Read the model definition and answer for the solid it produces. Units are mm, in the model's axes. A direction names the side the tool comes from. Coordinates: 2 decimals unless noted, no trailing zeros. Write each loop counter-clockwise with the first axis right and the second up, starting at its lowest first coordinate (ties: lowest second). Pieces come first, ordered by that corner, then holes.
(1) Section C-C on x = -11 is taken. Write down the section's boundary in (y, z) (3 decimals), then the cut area to 3 significant figures.
(2) Given pin 1 (6 mm diameter, centred on x = -8.5, z = 97.5, fed in from +Y); pin 2 (6 mm diameter, centred on y = 5.5, z = 62.5, fed in from -X); pin 3 (12 mm diameter, centred on x = -9.5, y = 12, fed in from +Z), each flat-ended and moving along its own axis, determine where each tip first touches the part or whether it passes through.
(3) Find the intervals of material crossed by probe 1 along Y at (x, z) = (-12.25, 98); probe 2 along X at (y, z) = (25.5, 218), in increasing order.
(4) Section A-A on z = 213.5 is taken. Write down the section's boundary in (x, y).
(5) Section D-D on y = 18 is taken. Write down the section's boundary in (x, z).
(6) Section B-B on z = 262 is taken. Write down the section's boundary in (x, y) (3 decimals), then the cut area to 3 significant figures.
(7) Which of the six approach directions +Z, -Z, +X, -X, +Y, -Y give full straight-line access (tool end or side, diameter ignored) to faces 1 (the flat face through (1, 6, 0)), 2 (the flat face through (0, 15, 169))?
from build123d import *

# Parameters (mm, degrees)
BASIS_BLECH1_DEPTH                          = 342
VERRUNDUNG1_R                               = 5
FORMSENKUNG_F_R_M5_SENKSCHRAUBE_MIT_2_COUNT = 2
FORMSENKUNG_F_R_M5_SENKSCHRAUBE_MIT_2_PITCH = 207


# Sheet-metal steps are written as plain solids
with BuildPart() as part:
    # Skizze1 → Basis-Blech1 (new body)
    with BuildSketch(Plane.XY):
        with BuildLine():
            Line((0, 30), (0, 0.1))
            ThreePointArc((0, 0.1), (-0.029289322, 0.029289322), (-0.1, 0))
            Line((-0.1, 0), (-20, 0))
            Line((-20, 0), (-20, -2))
            Line((-20, -2), (-0.1, -2))
            ThreePointArc((-0.1, -2), (1.38492424, -1.38492424), (2, 0.1))
            Line((2, 0.1), (2, 30))
            Line((2, 30), (0, 30))
        make_face()
    extrude(amount=BASIS_BLECH1_DEPTH)

    # Verrundung1
    verrundung1_edges = [part.edges().sort_by_distance(p)[0] for p in [
        (1, 30, 342),
        (1, 30, 0),
    ]]
    fillet(verrundung1_edges, radius=VERRUNDUNG1_R)

    # Skizze2 → Formsenkung für M5 Senkschraube mit Innensechskant1 (revolve, cut)
    with BuildSketch(Plane(origin=(-11, 0, 55), x_dir=(0, 0, 1), z_dir=(1, 0, 0))):
        Polygon((0, 0), (0, 2), (2.75, 2), (2.75, 2.985), (5.735, 0), align=None)
    formsenkung_f_r_m5_senkschraube_mit_inne = revolve(axis=Axis((-11, 6.35, 55), (0, -1, 0)), mode=Mode.SUBTRACT)

    # Formsenkung f_r M5 Senkschraube mit  2: Formsenkung für M5 Senkschraube mit Innensechskant1 ×2
    with Locations(*[(0, 0, i * FORMSENKUNG_F_R_M5_SENKSCHRAUBE_MIT_2_PITCH) for i in range(1, FORMSENKUNG_F_R_M5_SENKSCHRAUBE_MIT_2_COUNT)]):
        add(formsenkung_f_r_m5_senkschraube_mit_inne, mode=Mode.SUBTRACT)


solid = part.part
Response:
1. outline: (-2, 0) - (0, 0) - (0, 49.265) - (-2, 51.265) - close; (-2, 58.735) - (0, 60.735) - (0, 256.265) - (-2, 258.265) - close; (-2, 265.735) - (0, 267.735) - (0, 342) - (-2, 342) - close
1. area: 646 mm2
2. pin 1: stops at y = 0
2. pin 2: stops at x = 0
2. pin 3: passes through
3. probe 1: y = -2 to 0
3. probe 2: x = 0 to 2
4. outline: (-20, -2) - (-0.1, -2) arc R2.1 ccw to (2, 0.1) - (2, 30) - (0, 30) - (0, 0.1) arc R0.1 cw to (-0.1, 0) - (-20, 0) - close
5. outline: (0, 0) - (2, 0) - (2, 342) - (0, 342) - close
6. outline: (-20, -2) - (-14.735, -2) - (-16.735, 0) - (-20, 0) - close; (-7.265, -2) - (-0.1, -2) arc R2.1 ccw to (2, 0.1) - (2, 30) - (0, 30) - (0, 0.1) arc R0.1 cw to (-0.1, 0) - (-5.265, 0) - close
6. area: 84.1 mm2
7. face 1: -Z, +X, -X, +Y, -Y
7. face 2: +Z, -Z, -X, +Y
